from build123d import *

# Parameters (mm, degrees)
SKETCH_1_W          = 50
SKETCH_1_H          = 20
SKETCH_1_W_2        = 46
SKETCH_1_H_2        = 16
EXTRUDE_1_DEPTH     = 450
CUT_EXTRUDE_1_REACH = 454.88
SKETCH_2_R          = 3
CUT_EXTRUDE_2_REACH = 453.137
SKETCH_3_R          = 2


with BuildPart() as part:
    # Эскиз1 → Бобышка-Вытянуть1 (new body)
    with BuildSketch(Plane(origin=(0, 0, 0), x_dir=(0, 0, -1), z_dir=(1, 0, 0))):
        Rectangle(SKETCH_1_W, SKETCH_1_H)
        Rectangle(SKETCH_1_W_2, SKETCH_1_H_2, mode=Mode.SUBTRACT)
    extrude(amount=EXTRUDE_1_DEPTH)

    # Вырез-Вытянуть1: up to this face of the body (flat: up to its plane)
    cut_extrude_1_end = Plane(part.part.faces().sort_by_distance((225, 0, 25))[0])
    # Эскиз2 → Вырез-Вытянуть1 (cut, up to the picked face)
    with BuildSketch(Plane(origin=(0, 0, -25), x_dir=(-1, 0, 0), z_dir=(0, 0, -1)), mode=Mode.PRIVATE) as cut_extrude_1_sk1:
        with Locations((-415, 0)):
            Circle(SKETCH_2_R)
    cut_extrude_1_tool1 = split(extrude(cut_extrude_1_sk1.sketch, amount=-CUT_EXTRUDE_1_REACH, mode=Mode.PRIVATE), bisect_by=cut_extrude_1_end, keep=Keep.BOTH, mode=Mode.PRIVATE)
    # Эскиз2 → Вырез-Вытянуть1 (cut, up to the picked face)
    with BuildSketch(Plane(origin=(0, 0, -25), x_dir=(-1, 0, 0), z_dir=(0, 0, -1)), mode=Mode.PRIVATE) as cut_extrude_1_sk2:
        with Locations((-337.5, 0)):
            Circle(SKETCH_2_R)
    cut_extrude_1_tool2 = split(extrude(cut_extrude_1_sk2.sketch, amount=-CUT_EXTRUDE_1_REACH, mode=Mode.PRIVATE), bisect_by=cut_extrude_1_end, keep=Keep.BOTH, mode=Mode.PRIVATE)
    # Эскиз2 → Вырез-Вытянуть1 (cut, up to the picked face)
    with BuildSketch(Plane(origin=(0, 0, -25), x_dir=(-1, 0, 0), z_dir=(0, 0, -1)), mode=Mode.PRIVATE) as cut_extrude_1_sk3:
        with Locations((-112.5, 0)):
            Circle(SKETCH_2_R)
    cut_extrude_1_tool3 = split(extrude(cut_extrude_1_sk3.sketch, amount=-CUT_EXTRUDE_1_REACH, mode=Mode.PRIVATE), bisect_by=cut_extrude_1_end, keep=Keep.BOTH, mode=Mode.PRIVATE)
    # Эскиз2 → Вырез-Вытянуть1 (cut, up to the picked face)
    with BuildSketch(Plane(origin=(0, 0, -25), x_dir=(-1, 0, 0), z_dir=(0, 0, -1)), mode=Mode.PRIVATE) as cut_extrude_1_sk4:
        with Locations((-35, 0)):
            Circle(SKETCH_2_R)
    cut_extrude_1_tool4 = split(extrude(cut_extrude_1_sk4.sketch, amount=-CUT_EXTRUDE_1_REACH, mode=Mode.PRIVATE), bisect_by=cut_extrude_1_end, keep=Keep.BOTH, mode=Mode.PRIVATE)
    add(cut_extrude_1_tool1.solids().sort_by(Axis((415, 0, -25), (0, 0, 1)))[0], mode=Mode.SUBTRACT)
    add(cut_extrude_1_tool2.solids().sort_by(Axis((337.5, 0, -25), (0, 0, 1)))[0], mode=Mode.SUBTRACT)
    add(cut_extrude_1_tool3.solids().sort_by(Axis((112.5, 0, -25), (0, 0, 1)))[0], mode=Mode.SUBTRACT)
    add(cut_extrude_1_tool4.solids().sort_by(Axis((35, 0, -25), (0, 0, 1)))[0], mode=Mode.SUBTRACT)

    # Вырез-Вытянуть2: up to this face of the body (flat: up to its plane)
    cut_extrude_2_end = Plane(part.part.faces().sort_by_distance((225, -10, 0))[0])
    # Эскиз3 → Вырез-Вытянуть2 (cut, up to the picked face)
    with BuildSketch(Plane(origin=(0, 10, 0), x_dir=(1, 0, 0), z_dir=(0, 1, 0)), mode=Mode.PRIVATE) as cut_extrude_2_sk1:
        with Locations(Location((175, 0, 0), (0, 0, 270))):
            Circle(SKETCH_3_R)
    cut_extrude_2_tool1 = split(extrude(cut_extrude_2_sk1.sketch, amount=-CUT_EXTRUDE_2_REACH, mode=Mode.PRIVATE), bisect_by=cut_extrude_2_end, keep=Keep.BOTH, mode=Mode.PRIVATE)
    # Эскиз3 → Вырез-Вытянуть2 (cut, up to the picked face)
    with BuildSketch(Plane(origin=(0, 10, 0), x_dir=(1, 0, 0), z_dir=(0, 1, 0)), mode=Mode.PRIVATE) as cut_extrude_2_sk2:
        with Locations(Location((275, 0, 0), (0, 0, 270))):
            Circle(SKETCH_3_R)
    cut_extrude_2_tool2 = split(extrude(cut_extrude_2_sk2.sketch, amount=-CUT_EXTRUDE_2_REACH, mode=Mode.PRIVATE), bisect_by=cut_extrude_2_end, keep=Keep.BOTH, mode=Mode.PRIVATE)
    add(cut_extrude_2_tool1.solids().sort_by(Axis((175, 10, 0), (0, -1, 0)))[0], mode=Mode.SUBTRACT)
    add(cut_extrude_2_tool2.solids().sort_by(Axis((275, 10, 0), (0, -1, 0)))[0], mode=Mode.SUBTRACT)


solid = part.part
Work out the finished part from the listing and answer in its coordinate system (mm). A direction names the side the tool comes from. Coordinates: 2 decimals unless noted, no trailing zeros. Loops run counter-clockwise (first coordinate to the right, second up) from the corner with the lowest first, then second, coordinate; pieces in that order, holes last. Notation, with made-up numbers: (-36.5, -32.75) -> (-21.5, -32.75) arc R25 ccw to (-21.5, -4.75) -> close; hole circle Ø9 at (60, 10). An arc over 180 degrees is marked (long way). Write each question's results on one line, items separated by ' | '. Start each with the question number.
1) For faces 4 (the flat face through (0, 8.2, 0.1)), 5 (the flat face through (222, -8, 0)), determine the directions among +Z, -Z, +X, -X, +Y, -Y from which every point of the face is accessible in a straight line to the end or side of a thin tool.
2) Find section B-B on x = 287. Determine the outline of the cut face in (y, z).
3) The mould has two halves that part along Z. Classify faces 1 (the flat face through (222, 0, -25)), 2 (the flat face through (222, 8, 0)), 3 (the flat face through (222, 0, 25)): pulls with the +Z half, pulls with the -Z half, needs draft (parallel to the pull), parting line crosses it, or undercut.
4) A flat-ended cylindrical pin translates along its axis: P1, Ø4.5, axis at x = 175, z = 0, coming from the -Y side. Find the tip coordinate at first contact, or state that the pin passes through.
5) Find section A-A on z = 10.5. Determine the outline of the cut face in (x, y), then the cut area to 3 significant figures.
6) Consider line 1 along X through (y, z) = (9.1, 0); line 2 along Y through (x, z) = (86.5, -19); line 3 along Y through (x, z) = (415, -23.4). Determine where each line is inside the solid, lowest interval first.
Response values:
1) face 4: +Z, -Z, -X, +Y, -Y | face 5: +X, -X
2) outline: (-10, -25) -> (10, -25) -> (10, 25) -> (-10, 25) -> close; hole (-8, -23) -> (8, -23) -> (8, 23) -> (-8, 23) -> close
3) face 1: pulls with the -Z half | face 2: undercut | face 3: pulls with the +Z half
4) P1: stops at y = -10
5) outline: (0, -10) -> (450, -10) -> (450, -8) -> (0, -8) -> close; (0, 8) -> (450, 8) -> (450, 10) -> (0, 10) -> close | area: 1,800 mm^2
6) line 1: x = 0 to 173, 177 to 273, 277 to 450 | line 2: y = -10 to -8, 8 to 10 | line 3: y = -10 to -3, 3 to 10
